Can you work these out from the model? Positions are in its coordinate system, mm. A direction names the side the tool comes from. Round coordinates to 2 decimals unless told otherwise and drop trailing zeros. Order: outer loops, then holes, each group sorted by start corner. A loop starts at its lowest first (then second) coordinate and runs counter-clockwise, first axis right, second up.
Q1. Will these pins go through, and if not, where does the flat tip stop? P1, Ø23, axis at y = 371.5, z = 13.5, coming from the +X side; P2, Ø4, axis at y = -33.5, z = 3, coming from the +X side; P3, Ø6.5, axis at y = -41, z = 2.5, coming from the -X side.
Q2. If we section it at C-C (x = 267): Please give me the cut outline in (y, z).
Q3. If we section it at B-B (z = 16): Please give me the cut outline in (x, y), plus the area to 3 significant figures.
Q4. For faces 4 (the face through (-330.2, 288, -1)), 5 (the face through (355.6, 0, -1)), 6 (the face through (304.8, 276, 13)), which set-ups out of +Z, -Z, +X, -X, +Y, -Y let a thin tool reach every point of the face, with its end or its side?
Q5. We'd pull the mould along Y, two halves only. Please class faces 1 (the face through (-1, -55, 6.35)), 2 (the face through (5, 571.5, 1)), 3 (the face through (-161, 292.1, 12)): pulls with the +Y half, pulls with the -Y half, needs draft (parallel to the pull), parting line crosses it, or undercut.
Q6. If we section it at D-D (z = -41): Please give me the cut outline in (x, y), plus the area to 3 significant figures.
Q7. If we section it at A-A (x = 30): Please give me the cut outline in (y, z), plus the area to 3 significant figures.
Q8. If I drill on line 1 (X direction, y = 160, z = 22); line 2 (Y direction, x = -262, z = -10); line 3 (Y direction, x = 72.5, z = 40), over which ranges is the centre line in solid material (lowest first)?
from build123d import *

# Parameters (mm, degrees)
F0_W      = 711.2
F0_H      = 101.6
F1_DEPTH  = 12.7
F2_W      = 660.4
F2_H      = 101.6
F3_DEPTH  = 558.8
F4_W      = 609.6
F4_H      = 533.4
F5_DEPTH  = 76.2
F7_DEPTH  = 6.35
F9_W      = 292.1
F9_H      = 25.4
F10_DEPTH = 76.2


with BuildPart() as f1:
    # F0 (on Front) → F1 (new body, symmetric)
    with BuildSketch(Plane.XZ):
        Rectangle(F0_W, F0_H)
    extrude(amount=F1_DEPTH, both=True)

    # F2 (on face) → F3 (join)
    with BuildSketch(Plane(origin=(0, 12.7, 0), x_dir=(-1, 0, 0), z_dir=(0, 1, 0))):
        Rectangle(F2_W, F2_H)
    extrude(amount=F3_DEPTH)

    # F4 (on face) → F5 (cut)
    with BuildSketch(Plane.XY.offset(50.8)):
        with Locations((0, 279.4)):
            Rectangle(F4_W, F4_H)
    extrude(amount=-F5_DEPTH, mode=Mode.SUBTRACT)

    # F6 (on Top) → F7 (join, symmetric)
    with BuildSketch(Plane.XY):
        Polygon((-38.009446, -12.7), (-50.8, -12.7), (-50.8, -63.5), (50.8, -63.5), (50.8, -12.7), (38.1, -12.7), (38.1, -50.8), (-38.009446, -50.8), align=None)
    extrude(amount=F7_DEPTH, both=True)

    # F9 (on face) → F10 (join)
    with BuildSketch(Plane.XY.offset(-25.4)):
        with Locations((-158.75, 279.4)):
            Rectangle(F9_W, F9_H)
        Polygon((-12.7, 546.1), (-12.7, 292.1), (-12.7, 266.7), (-12.7, 12.7), (12.7, 12.7), (12.7, 546.1), align=None)
    extrude(amount=F10_DEPTH)


solid = f1.part
Solution:
1. P1: stops at x = 330.2
1. P2: stops at x = 50.8
1. P3: stops at x = -50.8
2. outline: (-12.7, -50.8) - (571.5, -50.8) - (571.5, 50.8) - (546.1, 50.8) - (546.1, -25.4) - (12.7, -25.4) - (12.7, 50.8) - (-12.7, 50.8) - close
3. outline: (-355.6, -12.7) - (355.6, -12.7) - (355.6, 12.7) - (330.2, 12.7) - (330.2, 571.5) - (-330.2, 571.5) - (-330.2, 12.7) - (-355.6, 12.7) - close; hole (-304.8, 12.7) - (-12.7, 12.7) - (-12.7, 266.7) - (-304.8, 266.7) - close; hole (-304.8, 292.1) - (-12.7, 292.1) - (-12.7, 546.1) - (-304.8, 546.1) - close; hole (12.7, 12.7) - (304.8, 12.7) - (304.8, 546.1) - (12.7, 546.1) - close
3. area: 82,900 mm2
4. face 4: +Z, -Z, -X, +Y
4. face 5: +Z, -Z, +X, +Y, -Y
4. face 6: +Z
5. face 1: needs draft
5. face 2: pulls with the +Y half
5. face 3: undercut
6. outline: (-355.6, -12.7) - (355.6, -12.7) - (355.6, 12.7) - (330.2, 12.7) - (330.2, 571.5) - (-330.2, 571.5) - (-330.2, 12.7) - (-355.6, 12.7) - close
6. area: 387,000 mm2
7. outline: (-63.5, -6.35) - (-50.8, -6.35) - (-50.8, 6.35) - (-63.5, 6.35) - close; (-12.7, -50.8) - (571.5, -50.8) - (571.5, 50.8) - (546.1, 50.8) - (546.1, -25.4) - (12.7, -25.4) - (12.7, 50.8) - (-12.7, 50.8) - close
7. area: 18,900 mm2
8. line 1: x = -330.2 to -304.8, -12.7 to 12.7, 304.8 to 330.2
8. line 2: y = -12.7 to 12.7, 266.7 to 292.1, 546.1 to 571.5
8. line 3: y = -12.7 to 12.7, 546.1 to 571.5
